Input: dimensioned drawing with shaded views. Units: mm. Origin: part minimum x, y, z. Coordinates: 2 decimals unless noted, no trailing zeros. Loops run counter-clockwise (first coordinate to the right, second up) from the corner with the lowest first, then second, coordinate; pieces in that order, holes last. Notation, with made-up numbers: (-37, -19.5) - (-1, -19.5) arc R13 ccw to (-1, -6.5) - close; hole circle Ø7 at (-22.75, 48.5). An arc over 180 degrees is marked (long way). Use one line per item in the form item = value. Start each with the question number.
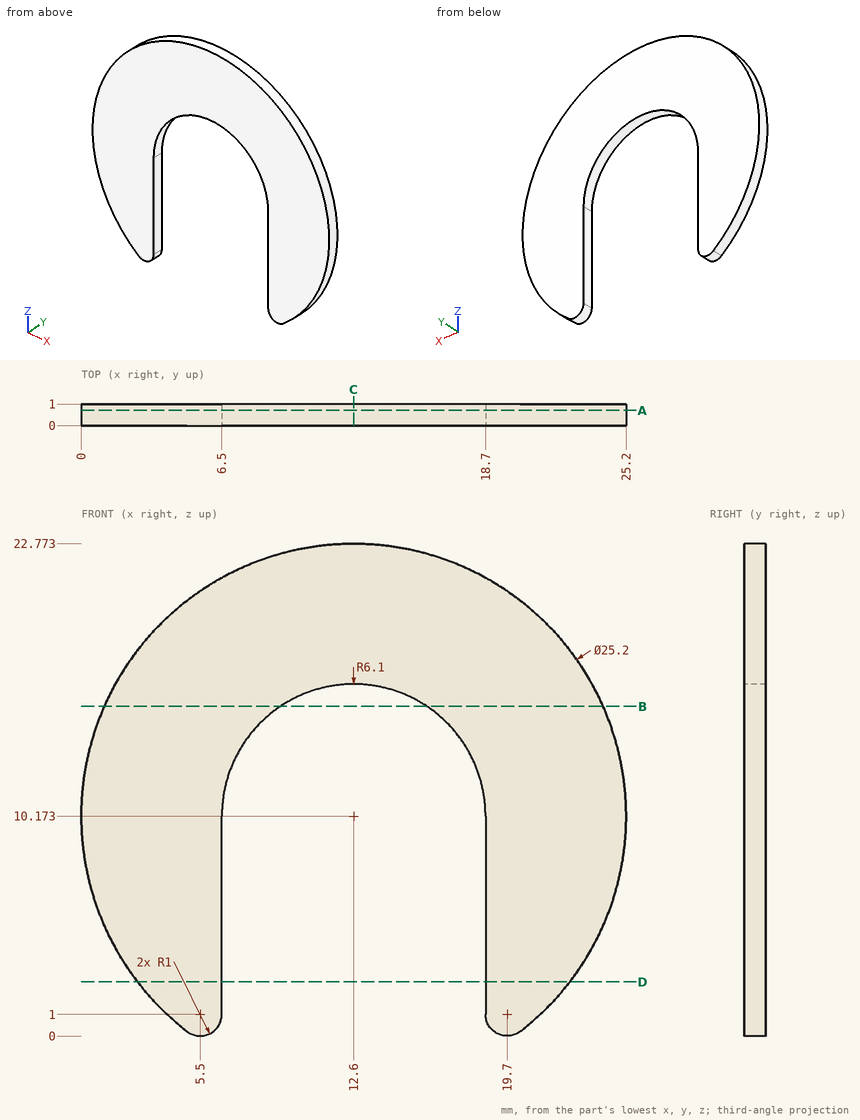
(1) Cut plane C-C, the plane x = 12.6. Output: boundary loops of the cut face in (y, z).
(2) Cut plane B-B, the plane z = 15.25. Output: boundary loops of the cut face in (x, y).
(3) Material intervals for line 1 (X direction, y = 0.7, z = 6.75); line 2 (X direction, y = 0.5, z = 12.75) (1 decimal); line 3 (Z direction, x = 6, y = 0.5) (1 decimal), sorted ascending.
(4) Cut plane A-A, the plane y = 0.7. Output: boundary loops of the cut face in (x, z).
(5) Contact query for a flat-ended pin moving along its axis: pin 1 (10 mm diameter, centred on x = 13, z = 9, fed in from -Y). Output: stop coordinate, or through.
(6) Cut plane D-D, the plane z = 2.5. Output: boundary loops of the cut face in (x, y).
Recorded:
q1.outline = (0, 16.27) - (1, 16.27) - (1, 22.77) - (0, 22.77) - close
q2.outline = (1.07, 0) - (9.22, 0) - (9.22, 1) - (1.07, 1) - close; (15.98, 0) - (24.13, 0) - (24.13, 1) - (15.98, 1) - close
q3.line_1 = 0.47 to 6.5, 18.7 to 24.73
q3.line_2 = 0.3 to 7.1, 18.1 to 24.9
q3.line_3 = 0.1 to 20.9
q4.outline = (4.89, 0.21) arc R1 ccw to (6.5, 1) - (6.5, 10.17) arc R6.1 cw to (18.7, 10.17) - (18.7, 1) arc R1 ccw to (20.31, 0.21) arc R12.6 ccw (long way) to start
q5.pin_1 = through
q6.outline = (2.61, 0) - (6.5, 0) - (6.5, 1) - (2.61, 1) - close; (18.7, 0) - (22.59, 0) - (22.59, 1) - (18.7, 1) - close
